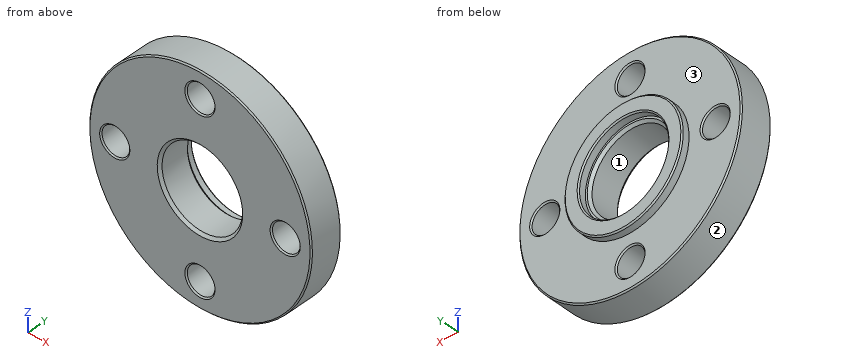
from build123d import *

# Parameters (mm, degrees)
CORTAR_EXTRUIR1_DEPTH      = 64.295931939
CORTAR_EXTRUIR1_DEPTH_BACK = 64.295931939
CROQUIS2_R                 = 5.5
CHAFL_N1_SIZE              = 1
CHAFL_N2_SIZE              = 0.5


with BuildPart() as part:
    # Croquis1 → Revolución1 (revolve)
    with BuildSketch(Plane(origin=(0, 0, 0), x_dir=(0, 0, -1), z_dir=(1, 0, 0))):
        Polygon((-16, -6.5), (-16, 6.5), (-17.75, 6.5), (-17.75, 9.5), (-23.5, 9.5), (-23.5, 6.5), (-44.25, 6.5), (-44.25, -6.5), align=None)
    revolve(axis=Axis((0, 0, 0), (0, -1, 0)))

    # Croquis2 → Cortar-Extruir1 (cut, two sides: drawn at the far end of the back side and taken through both)
    with BuildSketch(Plane(origin=(0, 0, 0), x_dir=(1, 0, 0), z_dir=(0, 1, 0)).offset(-CORTAR_EXTRUIR1_DEPTH_BACK)):
        with Locations(Location((0, 33.875, 0), (0, 0, 270))):
            Circle(CROQUIS2_R)
        with Locations(Location((33.875, 0, 0), (0, 0, 270))):
            Circle(CROQUIS2_R)
        with Locations(Location((0, -33.875, 0), (0, 0, 270))):
            Circle(CROQUIS2_R)
        with Locations(Location((-33.875, 0, 0), (0, 0, 270))):
            Circle(CROQUIS2_R)
    extrude(amount=CORTAR_EXTRUIR1_DEPTH + CORTAR_EXTRUIR1_DEPTH_BACK, mode=Mode.SUBTRACT)

    # Chaflán1
    chafl_n1_edges = [part.edges().sort_by_distance(p)[0] for p in [
        (0, 6.5, -16),
        (0, -6.5, -16),
    ]]
    chamfer(chafl_n1_edges, length=CHAFL_N1_SIZE)

    # Chaflán2
    chafl_n2_edges = [part.edges().sort_by_distance(p)[0] for p in [
        (0, 6.5, -39.375),
        (0, -6.5, -39.375),
        (33.875, 6.5, -5.5),
        (33.875, -6.5, -5.5),
        (0, 6.5, 28.375),
        (0, -6.5, 28.375),
        (-33.875, 6.5, -5.5),
        (-33.875, -6.5, -5.5),
        (0, -6.5, -44.25),
        (0, 6.5, -44.25),
        (0, 9.5, -23.5),
        (0, 9.5, -17.75),
    ]]
    chamfer(chafl_n2_edges, length=CHAFL_N2_SIZE)


solid = part.part
Model file for the job. Use its own axes, mm. Face numbers are marked on the shaded views. Coordinates: 2 decimals unless noted, no trailing zeros. Order: outer loops, then holes, each group sorted by start corner. A loop starts at its lowest first (then second) coordinate and runs counter-clockwise, first axis right, second up. Notation, with made-up numbers: (50, 80.25) -> (55, 80.25) arc R24 cw to (55, 101.25) -> close; hole circle Ø11 at (-30, -9). An arc over 180 degrees is marked (long way). Return JSON: item names as keys, results as strings. Group by question number.
Item 1: Flat gauge pins, fed straight in: P1, Ø5, axis at y = -0.5, z = 8, coming from the -X side; P2, Ø6, axis at y = -2, z = 3, coming from the -X side; P3, Ø1, axis at y = 1.5, z = -32, coming from the +X side; P4, Ø14.5, axis at x = 33.875, z = 0, coming from the -Y side. Where does each tip first touch, or does it go through?
Item 2: Pull direction X, two halves, no side cores. Call the marked faces 1, 2 and 3: pulls with the +X half, pulls with the -X half, needs draft (parallel to the pull), parting line crosses it, or undercut.
Item 3: Saw through at B-B on y = -1. Write the cut outline in (x, z) (3 decimals), then the cut area to 3 significant figures.
Item 4: Wall check: line 1 along X through (y, z) = (-1.75, 0) (3 decimals); line 2 along X through (y, z) = (7.1, 0). Give the ranges that are in metal, low to high. Write a range as [from, to].
Item 5: Saw through at A-A on x = 0. State how many separate pieces and enclosed holes the cut face has, then the cut area to 3 significant figures.
Values found:
{
 "1": {"P1": "stops at x = -43.91", "P2": "stops at x = -44.25", "P3": "stops at x = 31.08", "P4": "stops at y = -6.5"},
 "2": {"face 1": "undercut", "face 2": "parting line crosses it", "face 3": "needs draft"},
 "3": {"outline": "circle Ø88.5 at (0, 0); hole circle Ø11 at (-33.875, 0); hole circle Ø32 at (0, 0); hole circle Ø11 at (0, -33.875); hole circle Ø11 at (0, 33.875); hole circle Ø11 at (33.875, 0)", "area": "4,970 mm2"},
 "4": {"line 1": "x = [-44.25, -39.375], [-28.375, -16], [16, 28.375], [39.375, 44.25]", "line 2": "x = [-23.5, -17.75], [17.75, 23.5]"},
 "5": {"separate pieces": "4", "enclosed holes": "0", "area": "479 mm2"}
}
